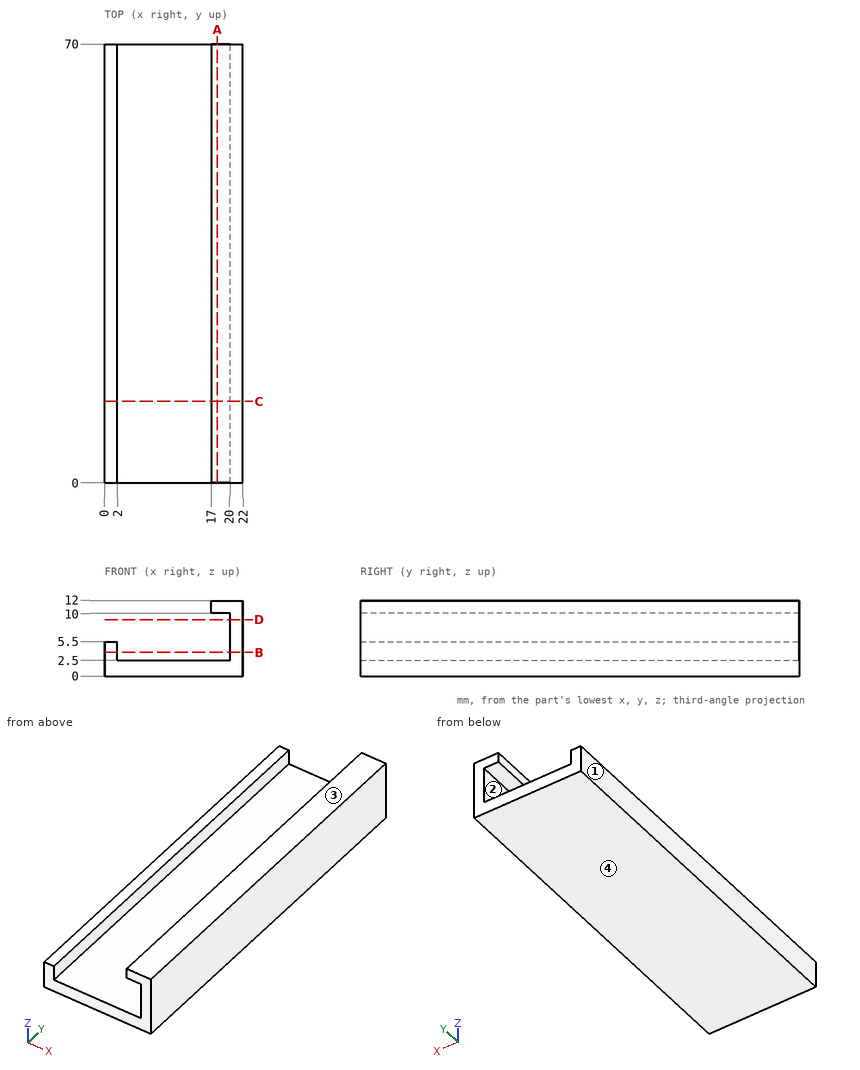
Drawing for the job (mm, zero at the part's lowest x, y, z). Coordinates: 2 decimals unless noted, no trailing zeros. Order: outer loops, then holes, each group sorted by start corner. A loop starts at its lowest first (then second) coordinate and runs counter-clockwise, first axis right, second up. Notation, with made-up numbers: (69.5, 17.25) -> (97.5, 17.25) arc R19 cw to (97.5, 36.25) -> close; hole circle Ø2 at (27.5, 68). An arc over 180 degrees is marked (long way). Answer in a Markdown table with one row per item.
1) Mould opens along Z. For the marked faces 1, 2, 3 and 4 say: pulls with the +Z half, pulls with the -Z half, needs draft (parallel to the pull), parting line crosses it, or undercut.
Check values:
| item | result |
|---|---|
| face 1 | needs draft |
| face 2 | undercut |
| face 3 | pulls with the +Z half |
| face 4 | pulls with the -Z half |
2) Flat gauge pins, fed straight in: P1, Ø1.5, axis at y = 39.5, z = 8, coming from the -X side; P2, Ø5, axis at x = 15, z = 6, coming from the -Y side; P3, Ø1, axis at y = 44, z = 11.5, coming from the -X side; P4, Ø1, axis at x = 3.5, y = 34, coming from the +Z side. Where does each tip first touch, or does it go through?
Check values:
| item | result |
|---|---|
| P1 | x = 20 |
| P2 | through |
| P3 | x = 17 |
| P4 | z = 2.5 |
3) Band-saw the part on C-C (y = 13). List the corners of the cut face in (x, z).
Check values:
| item | result |
|---|---|
| outline | (0, 0) -> (22, 0) -> (22, 12) -> (17, 12) -> (17, 10) -> (20, 10) -> (20, 2.5) -> (2, 2.5) -> (2, 5.5) -> (0, 5.5) -> close |
4) Band-saw the part on A-A (x = 18). List the corners of the cut face in (y, z).
Check values:
| item | result |
|---|---|
| outline | (0, 0) -> (70, 0) -> (70, 2.5) -> (0, 2.5) -> close; (0, 10) -> (70, 10) -> (70, 12) -> (0, 12) -> close |
5) Band-saw the part on D-D (z = 9). List the corners of the cut face in (x, y).
Check values:
| item | result |
|---|---|
| outline | (20, 0) -> (22, 0) -> (22, 70) -> (20, 70) -> close |
6) Band-saw the part on B-B (z = 3.75). List the corners of the cut face in (x, y).
Check values:
| item | result |
|---|---|
| outline | (0, 0) -> (2, 0) -> (2, 70) -> (0, 70) -> close; (20, 0) -> (22, 0) -> (22, 70) -> (20, 70) -> close |
7) Drill centre lines: line 1 (X direction, y = 28.5, z = 4.75); line 2 (Z direction, x = 19.5, y = 48); line 3 (Z direction, x = 11.25, y = 56). Where is each one in solid material? Low to high.
Check values:
| item | result |
|---|---|
| line 1 | 0 to 2, 20 to 22 |
| line 2 | 0 to 2.5, 10 to 12 |
| line 3 | 0 to 2.5 |
